Could you check a few things on this model? Use its own coordinates, in mm. Face numbers are marked on the shaded views. A direction names the side the tool comes from. Round coordinates to 2 decimals unless told otherwise and drop trailing zeros. Loops run counter-clockwise (first coordinate to the right, second up) from the corner with the lowest first, then second, coordinate; pieces in that order, holes last. Notation, with made-up numbers: (-23, -25.5) - (-7, -25.5) arc R22 ccw to (-7, -4.5) - close; hole circle Ø7 at (14.25, 50). An arc over 180 degrees is marked (long way). Put each result on its own line as item: value. Start each with the question number.
Autodesk Inventor part; units mm, degrees
ref_plane "YZ Plane" through (0, 0, 0) normal (1, 0, 0) x (0, 1, 0)
ref_plane "XZ Plane" through (0, 0, 0) normal (0, 1, 0) x (-1, 0, 0)
ref_plane "XY Plane" through (0, 0, 0) normal (0, 0, 1) x (1, 0, 0)
sketch "スケッチ1" plane through (0, 0, 0) normal (0, 0, 1) x (1, 0, 0)
  circle A0 centre (0, 0) radius 1.5
  dimension "d0" = 3
extrude "押し出し1" add sketch "スケッチ1" along normal blind 15
thread "ねじ1"
sketch "スケッチ2" plane through (0, 0, 15) normal (0, 0, 1) x (1, 0, 0)
  circle A0 centre (0, 0) radius 3
  dimension "d5" = 6
extrude "押し出し2" add sketch "スケッチ2" against normal blind 1.75
chamfer "面取り1" distance 1.5 angle 45 1 edges at (-3, 0, 13.25)
sketch "スケッチ3" plane through (0, 0, 15) normal (0, 0, 1) x (1, 0, 0)
  line L0 (0, 1.1547) -> (1, 0.5774)
  line L1 (1, 0.5774) -> (1, -0.5774)
  line L2 (1, -0.5774) -> (0, -1.1547)
  line L3 (0, -1.1547) -> (-1, -0.5774)
  line L4 (-1, -0.5774) -> (-1, 0.5774)
  line L5 (-1, 0.5774) -> (0, 1.1547)
  point P0 (0, 0)
  point P1 (0, 0)
  dimension "d11" = 2
extrude "押し出し3" cut sketch "スケッチ3" against normal blind 1.5
properties part number "m3皿ネジ15" material "鉄 灰色"
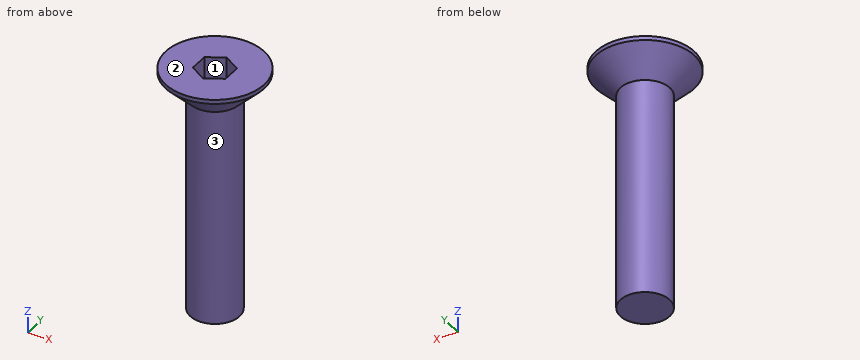
Item 1: I need wall thicknesses on line 1 (Y direction, x = -0.1, z = 7.75); line 2 (Y direction, x = 1, z = 11.5); line 3 (X direction, y = 0.35, z = 11.5). Which ranges of each line are inside material? Lowest first, please. Write a range as from..to.
Item 2: On a 3-axis mill with a long thin cutter (end or side, diameter ignored), from which of +Z, -Z, +X, -X, +Y, -Y can I reach the whole of each face in a straight line? I mean the marked faces 1, 2 and 3. Say none if no direction works.
Item 3: Will these pins go through, and if not, where does the flat tip stop? P1, Ø1.5, axis at x = -2, z = 11.5, coming from the +Y side; P2, Ø3, axis at x = 0.5, z = 2, coming from the +Y side; P3, Ø1.5, axis at y = 1, z = 11.5, coming from the +X side.
Item 4: Suppose I cut it at B-B, the plane z = 4.25. List the corners of the cut face in (x, y) for me.
Numbers:
1. line 1: -1.5..1.5
1. line 2: -1.12..1.12
1. line 3: -1.46..1.46
2. face 1: +Z
2. face 2: +Z, +X, -X, +Y, -Y
2. face 3: -Z
3. P1: y = 0.83
3. P2: y = 1.5
3. P3: x = 1.48
4. outline: circle Ø3 at (0, 0)
